Could you check a few things on this model? Use its own coordinates, in mm. A direction names the side the tool comes from. Coordinates: 2 decimals unless noted, no trailing zeros. Loops run counter-clockwise (first coordinate to the right, second up) from the corner with the lowest first, then second, coordinate; pieces in that order, holes last.
from build123d import *

# Parameters (mm, degrees)
EXTRUDE_1_DEPTH          = 362.5
CUT_EXTRUDE_2_DEPTH      = 433.557799606
CUT_EXTRUDE_2_DEPTH_BACK = 433.557799606
SKETCH_3_R               = 15.5


with BuildPart() as part:
    # 草图1 → 拉伸1 (new, symmetric)
    with BuildSketch(Plane.XY):
        Polygon((-174, 140), (-190, 140), (-190, -140), (-174, -140), (-174, -5), (174, -5), (174, -140), (190, -140), (190, 140), (174, 140), (174, 5), (-174, 5), align=None)
    extrude(amount=EXTRUDE_1_DEPTH, both=True)

    # 草图3 → 拉伸2 (cut, two sides: drawn at the far end of the back side and taken through both)
    with BuildSketch(Plane(origin=(0, 0, 0), x_dir=(0, 0, -1), z_dir=(1, 0, 0)).offset(-CUT_EXTRUDE_2_DEPTH_BACK)):
        with Locations((-312.5, 95)):
            Circle(SKETCH_3_R)
        with Locations((-212.5, 95)):
            Circle(SKETCH_3_R)
        with Locations((-112.5, 95)):
            Circle(SKETCH_3_R)
        with Locations(Location((-112.5, -95, 0), (0, 0, 270))):
            Circle(SKETCH_3_R)
        with Locations(Location((-212.5, -95, 0), (0, 0, 270))):
            Circle(SKETCH_3_R)
        with Locations(Location((-312.5, -95, 0), (0, 0, 270))):
            Circle(SKETCH_3_R)
        with Locations((312.5, -95)):
            Circle(SKETCH_3_R)
        with Locations((212.5, -95)):
            Circle(SKETCH_3_R)
        with Locations((112.5, -95)):
            Circle(SKETCH_3_R)
        with Locations(Location((112.5, 95, 0), (0, 0, 180))):
            Circle(SKETCH_3_R)
        with Locations(Location((212.5, 95, 0), (0, 0, 180))):
            Circle(SKETCH_3_R)
        with Locations(Location((312.5, 95, 0), (0, 0, 180))):
            Circle(SKETCH_3_R)
    extrude(amount=CUT_EXTRUDE_2_DEPTH + CUT_EXTRUDE_2_DEPTH_BACK, mode=Mode.SUBTRACT)


solid = part.part
(1) I need wall thicknesses on probe 1 along Y at (x, z) = (-180, 212); probe 2 along X at (y, z) = (63, 86); probe 3 along Y at (x, z) = (-63, 301). Which ranges of each line are inside material? Lowest first, please.
Answers:
probe 1: y = -140 to -110.49, -79.51 to 79.51, 110.49 to 140
probe 2: x = -190 to -174, 174 to 190
probe 3: y = -5 to 5
(2) Imagine slicing it at B-B, the plane z = -312.5. Write out the boundary of the cut face in (x, y).
Answers:
outline: (-190, -140) - (-174, -140) - (-174, -110.5) - (-190, -110.5) - close; (-190, -79.5) - (-174, -79.5) - (-174, -5) - (174, -5) - (174, -79.5) - (190, -79.5) - (190, 79.5) - (174, 79.5) - (174, 5) - (-174, 5) - (-174, 79.5) - (-190, 79.5) - close; (-190, 110.5) - (-174, 110.5) - (-174, 140) - (-190, 140) - close; (174, -140) - (190, -140) - (190, -110.5) - (174, -110.5) - close; (174, 110.5) - (190, 110.5) - (190, 140) - (174, 140) - close
(3) We'd pull the mould along Y, two halves only. Please class faces 1 (the face through (-182.112, -79.632, -210.482)), 2 (the face through (-2, -5, 5)), 3 (the face through (-174, -73, 5)): +Y half, -Y half, draft (parallel to the pull), parting line (faces both ways), or undercut.
Answers:
face 1: undercut
face 2: -Y half
face 3: draft
(4) Imagine slicing it at A-A, the plane y = -15.5. Write out the boundary of the cut face in (x, z), and give its area (3 significant figures).
Answers:
outline: (-190, -362.5) - (-174, -362.5) - (-174, 362.5) - (-190, 362.5) - close; (174, -362.5) - (190, -362.5) - (190, 362.5) - (174, 362.5) - close
area: 23,200 mm2
(5) Imagine slicing it at C-C, the plane y = 95. State how many separate pieces and enclosed holes the cut face has, and give its area (3 significant figures).
Answers:
separate pieces: 14
enclosed holes: 0
area: 17,200 mm2
(6) For pin 1 (6 mm diameter, centred on x = -52.5, z = -34, fed in from -Y); pin 2 (10 mm diameter, centred on x = -113.5, z = 131, fed in from +Y), each with a flat end and sliding along its axis, tell me the tip position at first contact or that it passes through.
Answers:
pin 1: stops at y = -5
pin 2: stops at y = 5
(7) Imagine slicing it at D-D, the plane x = 104. Write out the boundary of the cut face in (y, z), and give its area (3 significant figures).
Answers:
outline: (-5, -362.5) - (5, -362.5) - (5, 362.5) - (-5, 362.5) - close
area: 7,250 mm2
(8) Which directions (+Z, -Z, +X, -X, +Y, -Y) give clear straight access to the entire face, cutting with the end or side of a thin tool? Please do faces 4 (the face through (181.89, -82.7, 321.93)), 5 (the face through (2, 5, 5)).
Answers:
face 4: +X, -X
face 5: +Z, -Z, +Y
